Here's how the part is built. I have some questions about the finished solid (model axes, mm). A direction names the side the tool comes from. Give positions to 0.01 mm unless a question says otherwise; leave off trailing zeros. Write each loop counter-clockwise with the first axis right and the second up, starting at its lowest first coordinate (ties: lowest second). Pieces come first, ordered by that corner, then holes. Notation, with made-up numbers: (69, -10) -> (86, -10) arc R31 cw to (86, 15) -> close; hole circle Ø6 at (19, 30). An arc over 180 degrees is marked (long way). Use one line per item in the form item = value.
Autodesk Inventor part; units mm, degrees
ref_plane "YZ Plane" through (0, 0, 0) normal (1, 0, 0) x (0, 1, 0)
ref_plane "XZ Plane" through (0, 0, 0) normal (0, 1, 0) x (-1, 0, 0)
ref_plane "XY Plane" through (0, 0, 0) normal (0, 0, 1) x (1, 0, 0)
sketch "Sketch1" plane through (0, 0, 0) normal (0, 0, 1) x (1, 0, 0)
  line L0 (0, 0) -> (-190.3129, 0)
  line L1 (-190.3129, 0) -> (-190.3129, -1500)
  line L2 (-190.3129, -1500) -> (0, -1500)
  line L3 (0, -1500) -> (0, 0)
  line L4 (-190.3129, -1400) -> (-81, -1400)
  line L5 (-81, -1400) -> (-81, -1394)
  line L6 (-81, -1394) -> (-190.3129, -1394)
  line L7 (-190.3129, -1394) -> (-190.3129, -1400)
  line L8 (-190.3129, -900) -> (-81, -900)
  line L9 (-81, -900) -> (-81, -894)
  line L10 (-81, -894) -> (-190.3129, -894)
  line L11 (-190.3129, -894) -> (-190.3129, -900)
  line L12 (-190.3129, -400) -> (-81, -400)
  line L13 (-81, -400) -> (-81, -394)
  line L14 (-81, -394) -> (-190.3129, -394)
  line L15 (-190.3129, -394) -> (-190.3129, -400)
  point P0 (-190.3129, -400)
  point P1 (-190.3129, -894)
  point P2 (-190.3129, -900)
  dimension "d0" = 1500
  dimension "d1" = 190.3129
  dimension "d2" = 6
  dimension "d4" = 100
  dimension "d7" = 500
  dimension "d23" = 81
extrude "Plate1" add sketch "Sketch1" along normal blind 4 contours L3 L2 L1 L4 L5 L6 L8 L9 L10 L12 L13 L14 L0
sketch "Sketch2" plane through (4, 0, 0) normal (-1, 0, 0) x (0, -1, 0)
  line L0 (1500, 0) -> (0, 0)
  line L1 (0, 0) -> (0, 35)
  line L2 (0, 35) -> (1500, 35)
  line L3 (1500, 35) -> (1500, 0)
edge flange "Flange1" height 35 angle 90 thickness 4 bend radius 4 thickness toward (-1, 0, 0) relief tear relief width 4 relief depth 2 edges at (0, -750, 4) wall of the first edge with corners at (4, -1500, 0) (4, 0, 0) (4, 0, 35) (4, -1500, 35)
bend "Bend1"
corner "Corner1"
equation "\"d1\" = стрингерглубина1"
equation "\"d12\" = Thickness"
equation "\"d13\" = BendReliefWidth"
equation "\"d14\" = BendReliefDepth"
equation "\"d15\" = MinimumRemnant"
equation "\"d16\" = TransitionRadius"
equation "\"d19\" = BendRadius"
equation "\"d20\" = CornerReliefSize"
equation "\"d21\" = GapSize"
equation "\"d22\" = JacobiRadiusSize"
equation "\"BendRadius\" = Thickness"
equation "\"BendReliefWidth\" = Thickness"
equation "\"BendReliefDepth\" = 0.5 * Thickness"
equation "\"CornerReliefSize\" = 4 * Thickness"
equation "\"MinimumRemnant\" = 2 * Thickness"
equation "\"TransitionRadius\" = BendRadius"
equation "\"JacobiRadiusSize\" = BendRadius"
equation "\"GapSize\" = Thickness"
properties part number "stringer 1_CPY2"
Q1. I want a section at A-A, the plane x = -158.5. Write out the boundary of the cut face in (y, z), and give its area (3 significant figures).
Result set:
outline = (-1500, 0) -> (-1400, 0) -> (-1400, 4) -> (-1500, 4) -> close; (-1394, 0) -> (-900, 0) -> (-900, 4) -> (-1394, 4) -> close; (-894, 0) -> (-400, 0) -> (-400, 4) -> (-894, 4) -> close; (-394, 0) -> (0, 0) -> (0, 4) -> (-394, 4) -> close
area = 5,930 mm2
Q2. If we mould it in two halves opening along Z, with no side actions, what happens to faces 1 (the face through (-98, -740, 0)), 2 (the face through (-71, -1500, 3)), 3 (the face through (-98, -740, 4))? For each: +Z half, -Z half, draft (parallel to the pull), parting line (faces both ways), or undercut.
Result set:
face_1 = -Z half
face_2 = draft
face_3 = +Z half
Q3. Which directions (+Z, -Z, +X, -X, +Y, -Y) give clear straight access to the entire face, cutting with the end or side of a thin tool? Please do faces 4 (the face through (0, -740, 21)), 5 (the face through (4, -740, 22)).
Result set:
face_4 = +Z, -X, +Y, -Y
face_5 = +Z, -Z, +X, +Y, -Y
Q4. I want a section at B-B, the plane y = -803.5. Write out the boundary of the cut face in (x, z), and give its area (3 significant figures).
Result set:
outline = (-190.31, 0) -> (-4, 0) arc R8 ccw to (4, 8) -> (4, 35) -> (0, 35) -> (0, 8) arc R4 cw to (-4, 4) -> (-190.31, 4) -> close
area = 891 mm2
Q5. I want a section at D-D, the plane x = -26.5. Write out the boundary of the cut face in (y, z).
Result set:
outline = (-1500, 0) -> (0, 0) -> (0, 4) -> (-1500, 4) -> close
Q6. If I drill on line 1 along Z through (x, y) = (-132, -1064.5); line 2 along X through (y, z) = (-187.5, 6.5), over which ranges is the centre line in solid material (lowest first)? Write a range as from..to.
Result set:
line_1 = 0..4
line_2 = -0.29..3.86
Q7. Will these pins go through, and if not, where does the flat tip stop? pin 1 Ø2 at (x, z) = (-156.5, 1) entering from +Y; pin 2 Ø2 at (y, z) = (-397, 2) entering from -X; pin 3 Ø13.5 at (y, z) = (-841, 25) entering from -X; pin 4 Ø4 at (y, z) = (-307, 6.5) entering from -X.
Result set:
pin_1 = 0
pin_2 = -81
pin_3 = 0
pin_4 = -2.06
Q8. I want a section at C-C, the plane z = 18. Write out the boundary of the cut face in (x, y), and give its area (3 significant figures).
Result set:
outline = (0, -1500) -> (4, -1500) -> (4, 0) -> (0, 0) -> close
area = 6,000 mm2
